from build123d import *

# Parameters (mm, degrees)
F0_W      = 12.7
F0_H      = 12.7
F1_DEPTH  = 482.6
F2_R      = 3.175
F3_DEPTH  = 12.7
F4_R      = 3.175
F5_DEPTH  = 12.7
F6_W      = 12.7
F6_H      = 12.7
F7_DEPTH  = 6.35
F8_R      = 6.34999
F9_W      = 12.7
F9_H      = 12.7
F10_DEPTH = 6.35
F11_R     = 6.34999
F12_R     = 1.5875


# Not quite as in the source:
# - a fillet or chamfer is up to 0.001 mm smaller than in the source, because OpenCascade refuses the exact size


with BuildPart() as f1:
    # F0 (on Top) → F1 (new body)
    with BuildSketch(Plane.XY):
        with Locations((6.35, 6.35)):
            Rectangle(F0_W, F0_H)
    extrude(amount=-F1_DEPTH)

    # F2 (on face) → F3 (join)
    with BuildSketch(Plane.XY):
        with Locations((6.35, 6.35)):
            Circle(F2_R)
    extrude(amount=F3_DEPTH)

    # F4 (on face) → F5 (join)
    with BuildSketch(Plane(origin=(0, 0, -482.6), x_dir=(1, 0, 0), z_dir=(0, 0, -1))):
        with Locations((6.35, -6.35)):
            Circle(F4_R)
    extrude(amount=F5_DEPTH)

    # F6 (on face) → F7 (join)
    with BuildSketch(Plane.XY.offset(12.7)):
        with Locations((6.35, 6.35)):
            Rectangle(F6_W, F6_H)
    extrude(amount=F7_DEPTH)

    # F8 (radius 6.35 in the source; OpenCascade refuses exactly that, so slightly less here)
    f8_edges = [f1.edges().sort_by_distance(p)[0] for p in [
        (0, 6.35, 19.05),
        (6.35, 0, 19.05),
        (12.7, 6.35, 19.05),
        (6.35, 12.7, 19.05),
    ]]
    fillet(f8_edges, radius=F8_R)

    # F9 (on face) → F10 (join)
    with BuildSketch(Plane(origin=(0, 0, -495.3), x_dir=(1, 0, 0), z_dir=(0, 0, -1))):
        with Locations((6.35, -6.35)):
            Rectangle(F9_W, F9_H)
    extrude(amount=F10_DEPTH)

    # F11 (radius 6.35 in the source; OpenCascade refuses exactly that, so slightly less here)
    f11_edges = [f1.edges().sort_by_distance(p)[0] for p in [
        (6.35, 0, -501.65),
        (0, 6.35, -501.65),
        (6.35, 12.7, -501.65),
        (12.7, 6.35, -501.65),
    ]]
    fillet(f11_edges, radius=F11_R)

    # F12
    f12_edges = [f1.edges().sort_by_distance(p)[0] for p in [
        (0, 0, -241.3),
        (0, 12.7, -241.3),
        (12.7, 0, -241.3),
        (12.7, 12.7, -241.3),
    ]]
    fillet(f12_edges, radius=F12_R)


solid = f1.part
For this review, take the finished solid that the model builds, in its own axes (mm). A direction names the side the tool comes from. Round coordinates to 2 decimals unless told otherwise and drop trailing zeros. Put each result on its own line as item: value.
Q1. Machinability: for faces 1 (the flat face through (0, 6, -238)), 2 (the flat face through (3, 5, -495.3)), which of the approach directions +Z, -Z, +X, -X, +Y, -Y give a long, thin tool a straight path to every point of the face, cutting with its end or side? Answer none if there is none.
Determined:
face 1: +Z, -Z, -X, +Y, -Y
face 2: none
Q2. Clearance check with flat-ended pins moving along their axes: pin 1 Ø4 at (x, y) = (5, 3) entering from -Z; pin 2 Ø2 at (x, y) = (6.5, 7.5) entering from +Z; pin 3 Ø5 at (x, y) = (5, 1.5) entering from +Z. State where each tip first meets the part, or that it passes through.
Determined:
pin 1: stops at z = -501.5
pin 2: stops at z = 19.05
pin 3: stops at z = 18.6
Q3. To check wall thickness, follow L1, parallel to Z at x = 12, y = 1.5; L2, parallel to Z at x = 10.25, y = 7.25; L3, parallel to X at y = 11.5, z = -244. State the ranges of each line that lie inside material, in increasing order. Write a range as [from, to].
Determined:
L1: z = [-498.2, -495.3], [-482.6, 0], [12.7, 15.6]
L2: z = [-500.31, -495.3], [-482.6, 0], [12.7, 17.71]
L3: x = [0.05, 12.65]
